The listing builds one solid part. Answer for the finished solid, in the listing's coordinates (mm). Give positions to 0.01 mm unless a question says otherwise; leave off trailing zeros. Loops run counter-clockwise (first coordinate to the right, second up) from the corner with the lowest first, then second, coordinate; pieces in that order, holes last. Notation, with made-up numbers: M 63.5,7 L 91.5,7 A14 cw 91.5,27 Z; hole C 22,55 d3. An arc over 180 degrees is marked long. One line per item, written item: value. Start each with the question number.
Q1. A cutting plane is placed at D-D, the plane x = -169. Determine the outline of the cut face in (y, z).
Q2. A cutting plane is placed at B-B, the plane y = -2.2. State how many separate pieces and enclosed holes the cut face has, and give its area (3 significant figures).
Q3. A cutting plane is placed at C-C, the plane z = 90. Determine the outline of the cut face in (x, y), and give its area (3 significant figures).
Q4. Flat-ended cylindrical pins translate along their axes: pin 1 (20 mm diameter, centred on x = -90, z = 0, fed in from +Y); pin 2 (1 mm diameter, centred on y = -1, z = -19, fed in from +X). Find the tip coordinate at first contact, or state that the pin passes through.
Q5. Consider L1, parallel to Z at x = -27.5, y = -2.3; L2, parallel to Z at x = -124.5, y = -1.7; L3, parallel to Z at x = -90, y = -0.75. Determine where each line is inside the solid, lowest interval first.
Q6. A cutting plane is placed at A-A, the plane x = -90. Determine the outline of the cut face in (y, z), and give its area (3 significant figures).
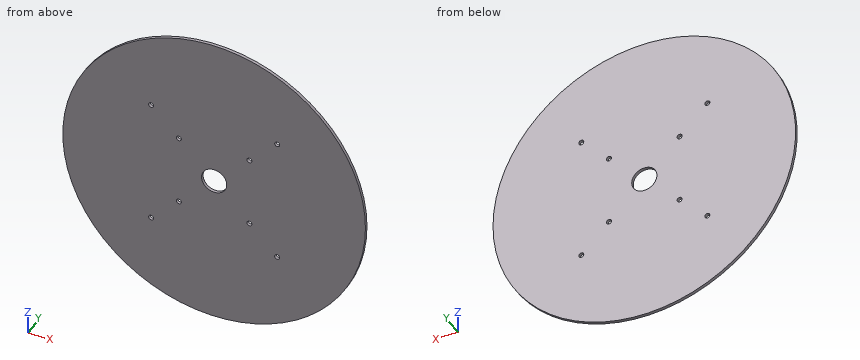
Autodesk Inventor part; units mm, degrees
ref_plane "YZ Plane" through (0, 0, 0) normal (1, 0, 0) x (0, 1, 0)
ref_plane "XZ Plane" through (0, 0, 0) normal (0, 1, 0) x (-1, 0, 0)
ref_plane "XY Plane" through (0, 0, 0) normal (0, 0, 1) x (1, 0, 0)
sketch "Sketch5" plane through (0, 0, -50) normal (0, -1, 0) x (1, 0, 0)
  line L0 (-90, 50) -> (35, 50) construction
  line L1 (60, 50) -> (-240, 50) construction
  line L2 (-180, 50) -> (0, 50) construction
  line L3 (0, 110) -> (0, -10) construction
  line L4 (-125, 85) -> (-55, 85) construction
  line L5 (-55, 85) -> (-55, 15) construction
  line L6 (-55, 15) -> (-125, 15) construction
  line L7 (-125, 15) -> (-125, 85) construction
  line L8 (-125, 85) -> (-55, 15) construction
  line L9 (-55, 85) -> (-125, 15) construction
  circle A0 centre (-90, 50) radius 150
  circle A1 centre (-125, 15) radius 2.5
  circle A2 centre (-55, 15) radius 2.5
  circle A3 centre (-55, 85) radius 2.5
  circle A4 centre (-125, 85) radius 2.5
  circle A5 centre (-90, 50) radius 12.5
  line L10 (-152.5, -12.5) -> (-27.5, -12.5) construction
  line L11 (-27.5, -12.5) -> (-27.5, 112.5) construction
  line L12 (-27.5, 112.5) -> (-152.5, 112.5) construction
  line L13 (-152.5, 112.5) -> (-152.5, -12.5) construction
  line L14 (-152.5, -12.5) -> (-27.5, 112.5) construction
  line L15 (-27.5, -12.5) -> (-152.5, 112.5) construction
  circle A6 centre (-152.5, -12.5) radius 2.5
  circle A7 centre (-27.5, -12.5) radius 2.5
  circle A8 centre (-27.5, 112.5) radius 2.5
  circle A9 centre (-152.5, 112.5) radius 2.5
  dimension "d57" = 300
  dimension "d25" = 125
  dimension "d50" = 70
  dimension "d51" = 70
  dimension "d52" = 5
  dimension "d53" = 25
  dimension "d54" = 125
  dimension "d55" = 125
  dimension "d56" = 5
extrude "Extrusion5" add sketch "Sketch5" along normal blind 3
properties part number "Foundation-Fork" material "Steel, Mild"
Answer block:
1. outline: M -3,-127.51 L 0,-127.51 L 0,127.51 L -3,127.51 Z
2. separate pieces: 1
2. enclosed holes: 9
2. area: 70,000 mm^2
3. outline: M -210,-3 L 30,-3 L 30,0 L -210,0 Z
3. area: 720 mm^2
4. pin 1: through
4. pin 2: x = 58.85
5. L1: -136.36 to -65, -60 to 60, 65 to 136.36
5. L2: -145.98 to -37.45, -32.55 to 32.55, 37.45 to 145.98
5. L3: -150 to -12.5, 12.5 to 150
6. outline: M -3,-150 L 0,-150 L 0,-12.5 L -3,-12.5 Z; M -3,12.5 L 0,12.5 L 0,150 L -3,150 Z
6. area: 825 mm^2
